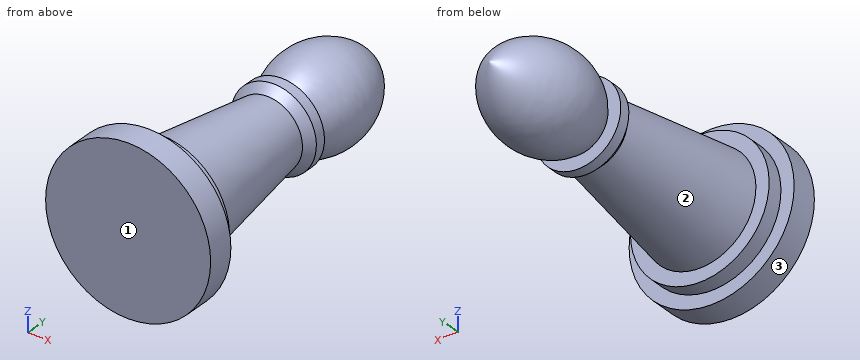
from build123d import *


with BuildPart() as part:
    # Sketch1 → Revolve1 (revolve)
    with BuildSketch(Plane.XY, mode=Mode.PRIVATE) as revolve1_sk:
        with BuildLine():
            Line((0, 0), (0, 38.1))
            ThreePointArc((0, 38.1), (-5.221326126, 31.976872569), (-3.437642592, 24.13))
            Line((-3.437642592, 24.13), (-4.919102977, 24.13))
            Line((-4.919102977, 24.13), (-4.919102977, 22.86))
            Line((-4.919102977, 22.86), (-4.0386, 21.873862293))
            Line((-4.0386, 21.873862293), (-6.477, 5.033662293))
            Line((-6.477, 5.033662293), (-8.001, 5.033662293))
            Line((-8.001, 5.033662293), (-8.001, 3.175))
            Line((-8.001, 3.175), (-9.525, 3.175))
            Line((-9.525, 3.175), (-9.525, 0))
            Line((-9.525, 0), (0, 0))
        make_face()
    revolve(revolve1_sk.sketch.rotate(Axis((0, 38.1, 0), (0, -1, 0)), 270), axis=Axis((0, 38.1, 0), (0, -1, 0)))


solid = part.part
Build history of the part. All positions in model axes, mm. Face numbers are marked on the shaded views. Round coordinates to 2 decimals unless told otherwise and drop trailing zeros. Write each loop counter-clockwise with the first axis right and the second up, starting at its lowest first coordinate (ties: lowest second). Pieces come first, ordered by that corner, then holes. Notation, with made-up numbers: M 18.5,-7.75 L 45.5,-7.75 A4 ccw 45.5,-1.75 Z; hole C 79.25,55 d9. An arc over 180 degrees is marked long. Answer as a JSON object with one key per item and string values. Group by question number.
(1) Cut at A-A (x = 7.5). Give the cut face in (y, z) (3 decimals).
(2) Cut at C-C (z = -4.25). Give the number of separate pieces and of enclosed holes in the cut face, and give its area (3 significant figures).
(3) Cut at B-B (z = 7.25). Give the cut face in (x, y) (3 decimals).
(4) Mould opens along Y. For the marked faces 1, 2 and 3 say: pulls with the +Y half, pulls with the -Y half, needs draft (parallel to the pull), parting line crosses it, or undercut.
(5) Flat gauge pins, fed straight in: pin 1 (1.5 mm diameter, centred on x = -1.5, y = 19.5, fed in from -Z); pin 2 (6 mm diameter, centred on x = -3, y = 17.5, fed in from +Z); pin 3 (10 mm diameter, centred on x = 4, y = 32.5, fed in from -Z). Where does each tip first touch, or does it go through?
(6) Drill centre lines: L1, parallel to Y at x = -6.5, z = 5 (3 decimals); L2, parallel to Y at x = -4, z = -6.25; L3, parallel to X at y = 29, z = 2.25. Where is each one in solid material? Low to high.
Responses:
{
 "1": {"outline": "M 0,-5.872 L 3.175,-5.872 L 3.175,-2.787 L 5.034,-2.787 L 5.034,2.787 L 3.175,2.787 L 3.175,5.872 L 0,5.872 Z"},
 "2": {"separate pieces": "3", "enclosed holes": "0", "area": "233 mm2"},
 "3": {"outline": "M -6.178,0 L 6.178,0 L 6.178,3.175 L 3.384,3.175 L 3.384,5.034 L -3.384,5.034 L -3.384,3.175 L -6.178,3.175 Z"},
 "4": {"face 1": "pulls with the -Y half", "face 2": "undercut", "face 3": "needs draft"},
 "5": {"pin 1": "stops at z = -4.36", "pin 2": "stops at z = 4.9", "pin 3": "stops at z = -5.48"},
 "6": {"L1": "y = 0 to 3.175", "L2": "y = 0 to 5.03", "L3": "x = -4.96 to 4.96"}
}
